```python
from build123d import *

# Parameters (mm, degrees)
SKETCH1_W           = 105.5
SKETCH1_H           = 22.8
BOSS_EXTRUDE1_DEPTH = 2.96
FILLET1_R           = 13
SKETCH2_R           = 2.5
CUT_EXTRUDE1_DEPTH  = 5.92
SKETCH3_R           = 5.15
CUT_EXTRUDE2_DEPTH  = 2
SKETCH4_W           = 75.1
SKETCH4_H           = 14.58
BOSS_EXTRUDE3_DEPTH = 2.48
FILLET2_R           = 5.25
SKETCH6_W           = 75
SKETCH6_H           = 14.59
BOSS_EXTRUDE4_DEPTH = 2.6
FILLET4_R           = 4.5
SKETCH7_R           = 5
BOSS_EXTRUDE5_DEPTH = 14.25


with BuildPart() as part:
    # Sketch1 → Boss-Extrude1 (new, symmetric)
    with BuildSketch(Plane(origin=(0, 0, 0), x_dir=(1, 0, 0), z_dir=(0, 1, 0))):
        Rectangle(SKETCH1_W, SKETCH1_H)
    extrude(amount=BOSS_EXTRUDE1_DEPTH, both=True)

    # Fillet1
    # the kernel refuses this fillet: 13 mm, written as the material it takes off along each edge
    with BuildSketch(Plane(origin=(-52.75, 35.46, -11.4), x_dir=(1, 0, 0), z_dir=(0, -1, 0)), Plane(origin=(52.75, -35.46, -11.4), x_dir=(-1, 0, 0), z_dir=(0, 1, 0))) as fillet1_piece_1:
        with BuildLine():
            CenterArc((FILLET1_R, FILLET1_R), FILLET1_R, 180, 90)
            Line((0, FILLET1_R), (0, 0))
            Line((0, 0), (FILLET1_R, 0))
        make_face()
    extrude(amount=70.92, mode=Mode.SUBTRACT)
    with BuildSketch(Plane(origin=(-52.75, 35.46, 11.4), x_dir=(1, 0, 0), z_dir=(0, -1, 0)), Plane(origin=(52.75, -35.46, 11.4), x_dir=(-1, 0, 0), z_dir=(0, 1, 0))) as fillet1_piece_2:
        with BuildLine():
            CenterArc((FILLET1_R, -FILLET1_R), FILLET1_R, 90, 90)
            Line((0, -FILLET1_R), (0, 0))
            Line((0, 0), (FILLET1_R, 0))
        make_face()
    extrude(amount=70.92, mode=Mode.SUBTRACT)

    # Sketch2 → Cut-Extrude1 (cut)
    with BuildSketch(Plane(origin=(0, 2.96, 0), x_dir=(1, 0, 0), z_dir=(0, 1, 0))):
        with Locations(Location((-45.151162738, 0, 0), (0, 0, 270))):
            Circle(SKETCH2_R)
        with Locations(Location((45.151162738, 0, 0), (0, 0, 270))):
            Circle(SKETCH2_R)
    extrude(amount=-CUT_EXTRUDE1_DEPTH, mode=Mode.SUBTRACT)

    # Sketch3 → Cut-Extrude2 (cut)
    with BuildSketch(Plane(origin=(0, 2.96, 0), x_dir=(1, 0, 0), z_dir=(0, 1, 0))):
        with Locations(Location((-45.151162738, 0, 0), (0, 0, 270))):
            Circle(SKETCH3_R)
        with Locations(Location((45.151162738, 0, 0), (0, 0, 270))):
            Circle(SKETCH3_R)
    extrude(amount=-CUT_EXTRUDE2_DEPTH, mode=Mode.SUBTRACT)

    # Sketch4 → Boss-Extrude3 (add)
    with BuildSketch(Plane(origin=(0, 2.96, 0), x_dir=(1, 0, 0), z_dir=(0, 1, 0))):
        Rectangle(SKETCH4_W, SKETCH4_H)
    extrude(amount=BOSS_EXTRUDE3_DEPTH)

    # Fillet2
    fillet2_edges = [part.edges().sort_by_distance(p)[0] for p in [
        (-37.55, 4.2, -7.29),
        (-37.55, 4.2, 7.29),
        (37.55, 4.2, 7.29),
        (37.55, 4.2, -7.29),
    ]]
    fillet(fillet2_edges, radius=FILLET2_R)

    # Sketch6 → Boss-Extrude4 (add)
    with BuildSketch(Plane(origin=(0, 5.44, 0), x_dir=(1, 0, 0), z_dir=(0, 1, 0))):
        Rectangle(SKETCH6_W, SKETCH6_H)
    extrude(amount=BOSS_EXTRUDE4_DEPTH)

    # Fillet4
    fillet4_edges = [part.edges().sort_by_distance(p)[0] for p in [
        (-37.5, 6.74, -7.295),
        (-37.5, 6.74, 7.295),
        (37.5, 6.74, 7.295),
        (37.5, 6.74, -7.295),
    ]]
    fillet(fillet4_edges, radius=FILLET4_R)

    # Sketch7 → Boss-Extrude5 (add)
    with BuildSketch(Plane(origin=(0, 8.04, 0), x_dir=(1, 0, 0), z_dir=(0, 1, 0))):
        with Locations(Location((-31.5, 0, 0), (0, 0, 90))):
            Circle(SKETCH7_R)
        with Locations(Location((-15.75, 0, 0), (0, 0, 90))):
            Circle(SKETCH7_R)
        with Locations(Location((0, 0, 0), (0, 0, 90))):
            Circle(SKETCH7_R)
        with Locations(Location((15.75, 0, 0), (0, 0, 90))):
            Circle(SKETCH7_R)
        with Locations(Location((31.5, 0, 0), (0, 0, 90))):
            Circle(SKETCH7_R)
    extrude(amount=BOSS_EXTRUDE5_DEPTH)


solid = part.part
```
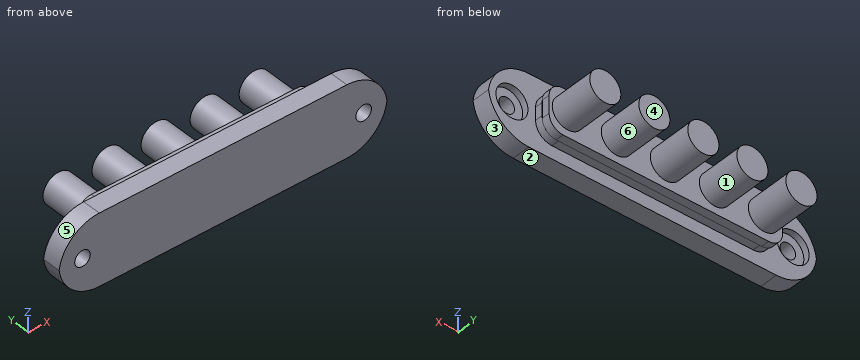
For this review, take the finished solid that the model builds, in its own axes (mm). Face numbers are marked on the shaded views. A direction names the side the tool comes from. Round coordinates to 2 decimals unless told otherwise and drop trailing zeros. Write each loop counter-clockwise with the first axis right and the second up, starting at its lowest first coordinate (ties: lowest second). Pieces come first, ordered by that corner, then holes.
1) Take a section at C-C on z = 6.25. Give the boundary of the cut face in (x, y).
Answer below:
outline: (-50.11, -2.96) - (50.11, -2.96) - (50.11, 2.96) - (35.44, 2.96) - (35.44, 5.44) - (35.88, 5.44) - (35.88, 8.04) - (-35.88, 8.04) - (-35.88, 5.44) - (-35.44, 5.44) - (-35.44, 2.96) - (-50.11, 2.96) - close
2) Take a section at A-A on y = 19. Give the boundary of the cut face in (x, z), then the cut area to 3 significant figures.
Answer below:
outline: circle Ø10 at (-31.5, 0); circle Ø10 at (-15.75, 0); circle Ø10 at (0, 0); circle Ø10 at (15.75, 0); circle Ø10 at (31.5, 0)
area: 393 mm2
3) Take a section at B-B on x = 0. Give the boundary of the cut face in (y, z) (3 decimals).
Answer below:
outline: (-2.96, -11.4) - (2.96, -11.4) - (2.96, -7.29) - (5.44, -7.29) - (5.44, -7.295) - (8.04, -7.295) - (8.04, -5) - (22.29, -5) - (22.29, 5) - (8.04, 5) - (8.04, 7.295) - (5.44, 7.295) - (5.44, 7.29) - (2.96, 7.29) - (2.96, 11.4) - (-2.96, 11.4) - close
4) Mouldability with a two-part tool opening along X and no side actions: class the marked faces 3, 4, 5 and 6 as +X half, -X half, draft (parallel to the pull), parting line (faces both ways), or undercut.
Answer below:
face 3: +X half
face 4: draft
face 5: -X half
face 6: undercut
5) Take a section at D-D on x = 41. Give the boundary of the cut face in (y, z), then the cut area to 3 significant figures.
Answer below:
outline: (-2.96, -11.34) - (2.96, -11.34) - (2.96, -3.05) - (0.96, -3.05) - (0.96, 3.05) - (2.96, 3.05) - (2.96, 11.34) - (-2.96, 11.34) - close
area: 122 mm2
6) Insertion check: pin 1 Ø11.5 at (x, z) = (44, -0.5) entering from +Y; pin 2 Ø3 at (y, z) = (6.5, 0) entering from -X; pin 3 Ø2.5 at (x, y) = (11.5, 4.5) entering from +Z (3 decimals); pin 4 Ø3 at (x, z) = (45.15, 0) entering from +Y. Each pin has a flat end and moves straight along its axis. Give the tip position at first contact, or say it passes through.
Answer below:
pin 1: stops at y = 2.96
pin 2: stops at x = -37.55
pin 3: stops at z = 7.295
pin 4: passes through
7) For line 1 along X through (y, z) = (19.25, -0.5); line 2 along Y through (x, z) = (-25, -0.75); line 3 along Y through (x, z) = (25, 9.5), list the stretches that pass through material, from the lowest coordinate up.
Answer below:
line 1: x = -36.47 to -26.53, -20.72 to -10.78, -4.97 to 4.97, 10.78 to 20.72, 26.53 to 36.47
line 2: y = -2.96 to 8.04
line 3: y = -2.96 to 2.96
8) Machinability: for the marked faces 1 and 2, which of the approach directions +Z, -Z, +X, -X, +Y, -Y give a long, thin tool a straight path to every point of the face, cutting with its end or side? Answer none if there is none.
Answer below:
face 1: +Y
face 2: -Z, +X, -X, +Y, -Y
